Design review of the part built by this model. Coordinates are the model's own, in mm. Face numbers are marked on the shaded views. Coordinates: 2 decimals unless noted, no trailing zeros. Order: outer loops, then holes, each group sorted by start corner. A loop starts at its lowest first (then second) coordinate and runs counter-clockwise, first axis right, second up. Notation, with made-up numbers: M 13,65 L 49,65 A15 cw 49,70 Z; hole C 67,1 d6. An arc over 180 degrees is marked long. Answer as a JSON object with one key per item and string values.
from build123d import *

# Parameters (mm, degrees)
SKETCH1_W      = 12.7
SKETCH1_H      = 25.4
EXTRUDE1_DEPTH = 12.7
SKETCH1_3_R    = 5.715
EXTRUDE2_DEPTH = 10.16
FILLET1_R      = 2.54


with BuildPart() as part:
    # Sketch1 → Extrude1 (new body)
    with BuildSketch(Plane.XY):
        Rectangle(SKETCH1_W, SKETCH1_H)
    extrude(amount=-EXTRUDE1_DEPTH)

    # Sketch1_3 → Extrude2 (add)
    with BuildSketch(Plane.XY):
        with Locations(Location((0, 0, 0), (0, 0, 180))):
            Circle(SKETCH1_3_R)
    extrude(amount=EXTRUDE2_DEPTH)

    # Sketch2 → Revolve1 (revolve)
    with BuildSketch(Plane(origin=(0, 0, 0), x_dir=(0, 0, -1), z_dir=(1, 0, 0)), mode=Mode.PRIVATE) as revolve1_sk:
        Polygon((-10.16, 1.016088838), (-24.491517392, -3.538898285), (-23.243143226, -6.1812071), (-10.16, 0), align=None)
    revolve(revolve1_sk.sketch.rotate(Axis((0, 0, 10.16), (0, -0.4271789944976144, 0.9041670789516765)), 180), axis=Axis((0, 0, 10.16), (0, -0.4271789944976144, 0.9041670789516765)))

    # Fillet1
    fillet1_edges = [part.edges().sort_by_distance(p)[0] for p in [
        (0, -3.538898285, 24.491517392),
    ]]
    fillet(fillet1_edges, radius=FILLET1_R)


solid = part.part
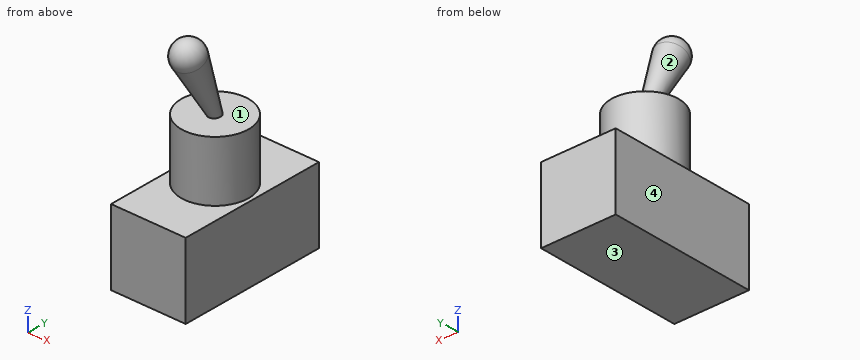
1) Add section C-C (y = 3.75). State the section outline as (x, z) points.
Taken from the geometry:
{"outline": "M -6.35,-12.7 L 6.35,-12.7 L 6.35,0 L 4.31,0 L 4.31,10.16 L -4.31,10.16 L -4.31,0 L -6.35,0 Z"}
2) To check wall thickness, follow L1, parallel to Z at x = 4.5, y = -7.5; L2, parallel to Z at x = -3.25, y = 2; L3, parallel to X at y = 2, z = 0.5. State the ranges of each line that lie inside material, in increasing order.
Taken from the geometry:
{"L1": "z = -12.7 to 0", "L2": "z = -12.7 to 10.16", "L3": "x = -5.35 to 5.35"}
3) Add section A-A (x = -3). State the section outline as (y, z) points, and give its area (3 significant figures).
Taken from the geometry:
{"outline": "M -12.7,-12.7 L 12.7,-12.7 L 12.7,0 L 4.86,0 L 4.86,10.16 L -4.86,10.16 L -4.86,0 L -12.7,0 Z", "area": "421 mm2"}
4) Mouldability with a two-part tool opening along Z and no side actions: class the marked faces 1, 2, 3 and 4 as released by +Z, released by -Z, zero draft, split by the parting line, or undercut.
Taken from the geometry:
{"face 1": "undercut", "face 2": "undercut", "face 3": "released by -Z", "face 4": "zero draft"}
5) Add section D-D (y = 8.25). State the section outline as (x, z) points.
Taken from the geometry:
{"outline": "M -6.35,-12.7 L 6.35,-12.7 L 6.35,0 L -6.35,0 Z"}
6) Insertion check: pin 1 Ø1.5 at (x, z) = (0.5, 19.5) entering from -Y; pin 2 Ø5 at (x, z) = (-5, 10.5) entering from +Y; pin 3 Ø3.5 at (x, y) = (1.5, -2.5) entering from +Z (3 decimals). Each pin has a flat end and moves straight along its axis. Give the tip position at first contact, or say it passes through.
Taken from the geometry:
{"pin 1": "stops at y = -7.53", "pin 2": "stops at y = 5.13", "pin 3": "stops at z = 23.175"}
7) Add section B-B (z = 9). State the section outline as (x, y) points (3 decimals).
Taken from the geometry:
{"outline": "C 0,0 d11.43"}
